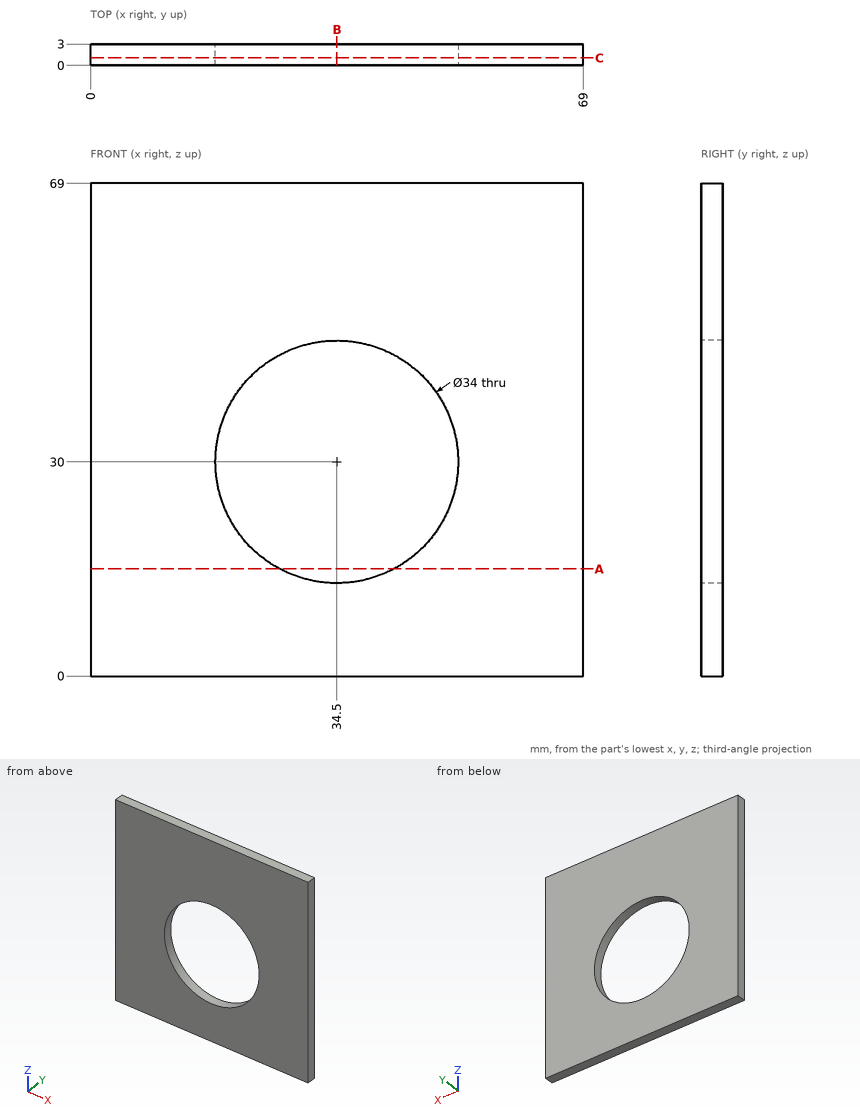
Source: three-view drawing plus pictorial views. Frame: mm from the lowest corner of the part. Round coordinates to 2 decimals unless told otherwise and drop trailing zeros. Loops run counter-clockwise (first coordinate to the right, second up) from the corner with the lowest first, then second, coordinate; pieces in that order, holes last.
Item 1: Section C-C, the plane y = 1.05. Output: boundary loops of the cut face in (x, z), plus the area to 3 significant figures.
Checked values:
outline: (0, 0) - (69, 0) - (69, 69) - (0, 69) - close; hole circle Ø34 at (34.5, 30)
area: 3,850 mm2
Item 2: Line query: L1, parallel to Z at x = 34.5, y = 1.95; L2, parallel to Z at x = 41, y = 1.85; L3, parallel to X at y = 0.25, z = 20. Output: solid intervals per line, ascending.
Checked values:
L1: z = 0 to 13, 47 to 69
L2: z = 0 to 14.29, 45.71 to 69
L3: x = 0 to 20.75, 48.25 to 69
Item 3: Section B-B, the plane x = 34.5. Output: boundary loops of the cut face in (y, z).
Checked values:
outline: (0, 0) - (3, 0) - (3, 13) - (0, 13) - close; (0, 47) - (3, 47) - (3, 69) - (0, 69) - close
Item 4: Section A-A, the plane z = 15. Output: boundary loops of the cut face in (x, y).
Checked values:
outline: (0, 0) - (26.5, 0) - (26.5, 3) - (0, 3) - close; (42.5, 0) - (69, 0) - (69, 3) - (42.5, 3) - close
